```python
from build123d import *

# Parameters (mm, degrees)
BOX002_W               = 140
BOX002_H               = 5
BOX002_DEPTH           = 250
BOX002_PLACEMENT_ANGLE = -45
CYLINDER_R             = 122
CYLINDER_DEPTH         = 20
CYLINDER_ROLL_ANGLE    = 90
BOX001_W               = 350
BOX001_H               = 64
BOX001_DEPTH           = 244
BOX_W                  = 350
BOX_H                  = 70
BOX_DEPTH              = 250


with BuildPart() as cube002:
    # Box002 → Box002 (new body)
    with BuildSketch(Plane.XY):
        with Locations((70, 2.5)):
            Rectangle(BOX002_W, BOX002_H)
    extrude(amount=BOX002_DEPTH)


with BuildPart() as cube002_1:
    # Box002 placement: moved
    add(cube002.part.moved(Location((172, 33, -125))).rotate(Axis((172, 33, -125), (0, 0, 1)), BOX002_PLACEMENT_ANGLE))


with BuildPart() as cylinder:
    # Cylinder → Cylinder (new body)
    with BuildSketch(Plane.XY):
        Circle(CYLINDER_R)
    extrude(amount=CYLINDER_DEPTH)


with BuildPart() as cylinder_1:
    # Cylinder roll: moved
    add(cylinder.part.rotate(Axis((0, 0, 0), (1, 0, 0)), CYLINDER_ROLL_ANGLE))


with BuildPart() as cylinder_2:
    # Cylinder placement: moved
    add(cylinder_1.part.moved(Location((175, -20, 0))))


with BuildPart() as cube001:
    # Box001 → Box001 (new body)
    with BuildSketch(Plane(origin=(-172, -32, -122), x_dir=(1, 0, 0), z_dir=(0, 0, 1))):
        with Locations((175, 32)):
            Rectangle(BOX001_W, BOX001_H)
    extrude(amount=BOX001_DEPTH)


with BuildPart() as fusion:
    # Box → Box (new body)
    with BuildSketch(Plane(origin=(-175, -35, -125), x_dir=(1, 0, 0), z_dir=(0, 0, 1))):
        with Locations((175, 35)):
            Rectangle(BOX_W, BOX_H)
    extrude(amount=BOX_DEPTH)

    # Cut: cut Cube001
    add(cube001.part, mode=Mode.SUBTRACT)

    # Cut001: cut Cylinder
    add(cylinder_2.part, mode=Mode.SUBTRACT)

    # Fusion: union Cube002
    add(cube002_1.part)


solid = fusion.part
```
Can you work these out from the model? Positions are in its coordinate system, mm. A direction names the side the tool comes from. Give positions to 0.01 mm unless a question says otherwise; leave off trailing zeros. Write each loop counter-clockwise with the first axis right and the second up, starting at its lowest first coordinate (ties: lowest second). Pieces come first, ordered by that corner, then holes. Notation, with made-up numbers: (49.25, -8.5) -> (104.25, -8.5) arc R21 ccw to (104.25, 6.5) -> close; hole circle Ø1 at (89.25, 30). An arc over 180 degrees is marked (long way). Write item = value, one per line.
(1) Suppose I cut it at D-D on x = 81.5. Write out the boundary of the cut face in (y, z), then the cut area to 3 significant figures.
Worked out:
outline = (-35, -125) -> (35, -125) -> (35, 125) -> (-35, 125) -> (-35, 78.37) -> (-32, 78.37) -> (-32, 122) -> (32, 122) -> (32, -122) -> (-32, -122) -> (-32, -78.37) -> (-35, -78.37) -> close
area = 1,410 mm^2
(2) I'm going to push flat-ended pins straight in: P1, Ø12, axis at x = -92.5, z = 0, coming from the -Y side; P2, Ø3.5, axis at y = 6, z = 124, coming from the +X side; P3, Ø0.9, axis at y = -11, z = -123.5, coming from the +X side; P4, Ø12, axis at x = -82, y = -46, coming from the -Z side. Where does each tip first touch, or does it pass through?
Worked out:
P1 = -35
P2 = 207.82
P3 = 223.52
P4 = through
(3) Suppose I cut it at A-A on x = 12.5. Write out the boundary of the cut face in (y, z), then the cut area to 3 significant figures.
Worked out:
outline = (-35, -125) -> (35, -125) -> (35, 125) -> (-35, 125) -> close; hole (-32, -122) -> (32, -122) -> (32, 122) -> (-32, 122) -> close
area = 1,880 mm^2
(4) For faces 4 (the face through (-3, 35, -2)), 5 (the face through (-39, -32, -2)), 6 (the face through (53.03, -33.48, 2.68)), 7 (the face through (-41, -35, -2)), which set-ups out of +Z, -Z, +X, -X, +Y, -Y let a thin tool reach every point of the face, with its end or its side?
Worked out:
face_4 = +Z, -Z, -X, +Y
face_5 = none
face_6 = -Y
face_7 = +Z, -Z, -X, -Y
(5) Suppose I cut it at B-B on y = 2. Write out the boundary of the cut face in (x, z).
Worked out:
outline = (-175, -125) -> (175, -125) -> (175, -122) -> (-172, -122) -> (-172, 122) -> (175, 122) -> (175, 125) -> (-175, 125) -> close; (203, -125) -> (210.07, -125) -> (210.07, 125) -> (203, 125) -> close
(6) Thinking about a two-plate mould opening in Z: for faces 1 (the face through (20, -2, 125)), 2 (the face through (-1, 0, 122)), 3 (the face through (224.34, -12.27, -1.75)), which applies, released by +Z, released by -Z, zero draft, split by the parting line, or undercut?
Worked out:
face_1 = released by +Z
face_2 = undercut
face_3 = zero draft
(7) I need wall thicknesses on probe 1 along Z at (x, y) = (-154.5, 12.5); probe 2 along Y at (x, z) = (-155, -10.5); probe 3 along Y at (x, z) = (159, -49). Which ranges of each line are inside material? Lowest first, please. Write a range as from..to.
Worked out:
probe_1 = -125..-122, 122..125
probe_2 = -35..-32, 32..35
probe_3 = 32..35
(8) Suppose I cut it at C-C on z = 0. Write out the boundary of the cut face in (x, y).
Worked out:
outline = (-175, -35) -> (53, -35) -> (53, -32) -> (-172, -32) -> (-172, 32) -> (173, 32) -> (270.99, -65.99) -> (274.53, -62.46) -> (175.54, 36.54) -> (174, 35) -> (-175, 35) -> close
